The model under review builds one solid part; all positions refer to its coordinate system, in mm. A direction names the side the tool comes from. Coordinates: 2 decimals unless noted, no trailing zeros. Write each loop counter-clockwise with the first axis right and the second up, starting at its lowest first coordinate (ties: lowest second). Pieces come first, ordered by that corner, then holes.
1) Add section A-A, the plane x = 8. State the section outline as (y, z) points.
2) Machinability: for faces 4 (the cylindrical face through (2.38, 13.43, -19.4)), 5 (the flat face through (3, 12, -7)), which of the approach directions +Z, -Z, +X, -X, +Y, -Y give a long, thin tool a straight path to every point of the face, cutting with its end or side? Answer none if there is none.
3) Add section B-B, the plane z = -10. State the section outline as (x, y) points.
4) Add section D-D, the plane z = -15. State the section outline as (x, y) points.
5) For P1, Ø3.5, axis at x = 10, z = -13, coming from the +Y side; P2, Ø3, axis at x = 5, z = -10, coming from the +Y side, all flat-tipped, find the tip position at first contact; note any pin that passes through.
6) For line 1 (Z direction, x = 10.5, y = 4.5); line 2 (X direction, y = 0.3, z = -10); line 3 (Z direction, x = 8, y = 0.4), list the stretches that pass through material, from the lowest coordinate up.
7) Mouldability with a two-part tool opening along X and no side actions: class faces 1 (the conical face through (7.9, 0.7, -12.4)), 2 (the flat face through (2, 14, -10)), 3 (the flat face through (9, 9, -1)) as released by +X, released by -X, zero draft, split by the parting line, or undercut.
from build123d import *

# Parameters (mm, degrees)
BOSS_EXTRUDE2_DEPTH = 20
SHELL1_START        = 3
SHELL1_OUTLINE_W    = 11
SHELL1_OUTLINE_H    = 14
SHELL1_DEPTH        = 11
FILLET3_R           = 2


# Read off the part's stored shape, not the designer's step: Shell1
with BuildPart() as part:
    # Sketch1 → Boss-Extrude2 (new body)
    with BuildSketch(Plane.XY):
        Polygon((0, 0), (0, 14), (4, 14), (14, 4), (14, 0), align=None)
    extrude(amount=-BOSS_EXTRUDE2_DEPTH)

    # Shell1 outline → Shell1 (cut)
    with BuildSketch(Plane(origin=(0, 0, 0), x_dir=(1, 0, 0), z_dir=(0, 1, 0)).offset(SHELL1_START)):
        with Locations((8.5, 10)):
            Rectangle(SHELL1_OUTLINE_W, SHELL1_OUTLINE_H)
    extrude(amount=SHELL1_DEPTH, mode=Mode.SUBTRACT)

    # Fillet3
    fillet3_edges = [part.edges().sort_by_distance(p)[0] for p in [
        (2, 14, -20),
        (2, 14, 0),
        (14, 2, 0),
        (14, 2, -20),
    ]]
    fillet(fillet3_edges, radius=FILLET3_R)

    # Sketch6 → CSK for M4 Flat Head Machine Screw3 (revolve, cut)
    with BuildSketch(Plane(origin=(3, 8, -10), x_dir=(0, 0, -1), z_dir=(0, 1, 0))):
        Polygon((0, 0), (0, 3), (2.25, 3), (2.25, 2.45), (4.7, 0), align=None)
    revolve(axis=Axis((9.35, 8, -10), (-1, 0, 0)), mode=Mode.SUBTRACT)

    # Sketch9 → CSK for M4 Flat Head Machine Screw2 (revolve, cut)
    with BuildSketch(Plane(origin=(8, 3, -10), x_dir=(0, 0, 1), z_dir=(1, 0, 0))):
        Polygon((0, 0), (0, 3), (2.25, 3), (2.25, 2.45), (4.7, 0), align=None)
    revolve(axis=Axis((8, 9.35, -10), (0, -1, 0)), mode=Mode.SUBTRACT)


solid = part.part
Geometry results:
1. outline: (0, -20) - (10, -20) - (10, -17) - (3, -17) - (3, -14.7) - (0.55, -12.25) - (0, -12.25) - close; (0, -7.75) - (0.55, -7.75) - (3, -5.3) - (3, -3) - (10, -3) - (10, 0) - (0, 0) - close
2. face 4: -Z, +X, -X, +Y
2. face 5: +X, +Y
3. outline: (0, 0) - (5.75, 0) - (5.75, 0.55) - (3.3, 3) - (3, 3) - (3, 3.3) - (0.55, 5.75) - (0, 5.75) - close; (0, 10.25) - (0.55, 10.25) - (3, 12.7) - (3, 14) - (0, 14) - close; (10.25, 0) - (14, 0) - (14, 3) - (12.7, 3) - (10.25, 0.55) - close
4. outline: (0, 0) - (14, 0) - (14, 3) - (3, 3) - (3, 14) - (0, 14) - close
5. P1: stops at y = 3
5. P2: stops at y = 2.8
6. line 1: z = -20 to -17, -3 to 0
6. line 2: x = 0 to 5.75, 10.25 to 14
6. line 3: z = -20 to -12.25, -7.75 to 0
7. face 1: undercut
7. face 2: zero draft
7. face 3: released by +X
